Can you work these out from the model? Positions are in its coordinate system, mm. A direction names the side the tool comes from. Coordinates: 2 decimals unless noted, no trailing zeros. Order: outer loops, then holes, each group sorted by start corner. A loop starts at its lowest first (then second) coordinate and runs counter-clockwise, first axis right, second up. Notation, with made-up numbers: (0.25, 20.5) -> (54.25, 20.5) arc R22 ccw to (54.25, 36.5) -> close; hole circle Ø9 at (58, 62). An arc over 180 degrees is marked (long way). Write item = value, one per line.
```python
from build123d import *

# Parameters (mm, degrees)
F1_DEPTH = 7.56
F2_T     = -3


with BuildPart() as f1:
    # F0 (on Top) → F1 (new body)
    with BuildSketch(Plane.XY):
        Polygon((41.38, 18.59), (0, 33.4360361274), (-41.38, 18.59), (-41.38, 0), (-55.43, -6.9778825002), (-53.92, -22.3639638726), (0, -22.3639638726), (53.92, -22.3639638726), (55.43, -6.9778825002), (41.38, 0), align=None)
    extrude(amount=F1_DEPTH)

    # F2
    f2_openings = [f1.faces().sort_by_distance(p)[0] for p in [
        (0, 0.369388, 7.56),
    ]]
    offset(amount=F2_T, openings=f2_openings, kind=Kind.INTERSECTION)


solid = f1.part
```
Item 1: I want a section at C-C, the plane z = 1. Please give me the cut outline in (x, y), plus the area to 3 significant figures.
A:
outline = (-55.43, -6.98) -> (-53.92, -22.36) -> (53.92, -22.36) -> (55.43, -6.98) -> (41.38, 0) -> (41.38, 18.59) -> (0, 33.44) -> (-41.38, 18.59) -> (-41.38, 0) -> close
area = 4,510 mm2
Item 2: I'm going to push flat-ended pins straight in: P1, Ø3.5, axis at x = -1, z = 5, coming from the +Y side; P2, Ø3, axis at y = -13.5, z = 2.5, coming from the -X side; P3, Ø4, axis at x = 8, z = 1.5, coming from the +Y side; P4, Ø3, axis at x = -9.5, z = 3.5, coming from the +Y side. Where does each tip first touch, or does it pass through?
A:
P1 = 33.44
P2 = -54.94
P3 = 31.28
P4 = 30.57
Item 3: I want a section at D-D, the plane x = 22. Please give me the cut outline in (y, z), plus the area to 3 significant figures.
A:
outline = (-22.36, 0) -> (25.54, 0) -> (25.54, 7.56) -> (22.36, 7.56) -> (22.36, 3) -> (-19.36, 3) -> (-19.36, 7.56) -> (-22.36, 7.56) -> close
area = 172 mm2
Item 4: For faces 4 (the flat face through (-41.38, 9, 4)), 5 (the flat face through (-51.73, -13.98, 5.25)), 6 (the flat face through (-54.686, -14.563, 3.727)), which set-ups out of +Z, -Z, +X, -X, +Y, -Y let a thin tool reach every point of the face, with its end or its side?
A:
face_4 = +Z, -Z, -X, +Y
face_5 = +Z
face_6 = +Z, -Z, -X, -Y
Item 5: I want a section at A-A, the plane z = 5.5. Please give me the cut outline in (x, y).
A:
outline = (-55.43, -6.98) -> (-53.92, -22.36) -> (53.92, -22.36) -> (55.43, -6.98) -> (41.38, 0) -> (41.38, 18.59) -> (0, 33.44) -> (-41.38, 18.59) -> (-41.38, 0) -> close; hole (-52.24, -8.74) -> (-51.2, -19.36) -> (51.2, -19.36) -> (52.24, -8.74) -> (38.38, -1.86) -> (38.38, 16.48) -> (0, 30.25) -> (-38.38, 16.48) -> (-38.38, -1.86) -> close
Item 6: I want a section at B-B, the plane y = 5. Please give me the cut outline in (x, z), plus the area to 3 significant figures.
A:
outline = (-41.38, 0) -> (41.38, 0) -> (41.38, 7.56) -> (38.38, 7.56) -> (38.38, 3) -> (-38.38, 3) -> (-38.38, 7.56) -> (-41.38, 7.56) -> close
area = 276 mm2
Item 7: If we mould it in two halves opening along Z, with no side actions, what happens to faces 1 (the flat face through (-1, 0, 0)), 2 (the flat face through (54.664, -14.779, 3.727)), 3 (the flat face through (-1, 0, 3))? For each: pulls with the +Z half, pulls with the -Z half, needs draft (parallel to the pull), parting line crosses it, or undercut.
A:
face_1 = pulls with the -Z half
face_2 = needs draft
face_3 = pulls with the +Z half
Item 8: If I drill on probe 1 along X at (y, z) = (11.5, 5.5); probe 2 along Z at (x, y) = (13.5, 17); probe 3 along Y at (x, z) = (33.5, 4), over which ranges is the centre line in solid material (lowest first)?
A:
probe_1 = -41.38 to -38.38, 38.38 to 41.38
probe_2 = 0 to 3
probe_3 = -22.36 to -19.36, 18.23 to 21.42
